```python
from build123d import *

# Parameters (mm, degrees)
F0_W     = 42
F0_H     = 17.5
F0_W_2   = 36
F0_H_2   = 11.5
F1_DEPTH = 40
F2_DEPTH = 3
F3_R     = 3
F4_R     = 2.99999


# Not quite as in the source:
# - a fillet or chamfer is up to 0.001 mm smaller than in the source, because OpenCascade refuses the exact size


with BuildPart() as f1:
    # F0 (on Top) → F1 (new body)
    with BuildSketch(Plane.XY):
        with Locations((12.1359585822, -3.1205574796)):
            Rectangle(F0_W, F0_H)
        with Locations((12.1359585822, -3.1205574796)):
            Rectangle(F0_W_2, F0_H_2, mode=Mode.SUBTRACT)
    extrude(amount=F1_DEPTH)

    # F0 (on Top) → F2 (join)
    with BuildSketch(Plane.XY):
        with Locations((12.1359585822, -3.1205574796)):
            Rectangle(F0_W, F0_H)
        with Locations((12.1359585822, -3.1205574796)):
            Rectangle(F0_W_2, F0_H_2, mode=Mode.SUBTRACT)
        with Locations((12.1359585822, -3.1205574796)):
            Rectangle(F0_W_2, F0_H_2)
    extrude(amount=-F2_DEPTH)

    # F3
    f3_edges = [f1.edges().sort_by_distance(p)[0] for p in [
        (33.135959, -11.870557, 18.5),
        (12.135959, -11.870557, -3),
        (33.135959, -3.120557, -3),
        (33.135959, 5.629443, 18.5),
        (12.135959, 5.629443, -3),
        (-8.864041, 5.629443, 18.5),
        (-8.864041, -3.120557, -3),
        (-8.864041, -11.870557, 18.5),
    ]]
    fillet(f3_edges, radius=F3_R)

    # F4 (radius 3 in the source; OpenCascade refuses exactly that, so slightly less here)
    f4_edges = [f1.edges().sort_by_distance(p)[0] for p in [
        (12.135959, 5.629443, 40),
        (-8.864041, -3.120557, 40),
        (12.135959, -11.870557, 40),
        (33.135959, -3.120557, 40),
    ]]
    fillet(f4_edges, radius=F4_R)


solid = f1.part
```
Can you work these out from the model? Positions are in its coordinate system, mm. A direction names the side the tool comes from. Coordinates: 2 decimals unless noted, no trailing zeros. Order: outer loops, then holes, each group sorted by start corner. A loop starts at its lowest first (then second) coordinate and runs counter-clockwise, first axis right, second up. Notation, with made-up numbers: (-32, 79.25) - (25, 79.25) arc R28 cw to (25, 116.25) - close; hole circle Ø10 at (59, -6.5). An arc over 180 degrees is marked (long way). Answer in a Markdown table with one row per item.
1. Suppose I cut it at A-A (z = 10.5). Please give me the cut outline in (x, y).
Reply:
| item | result |
|---|---|
| outline | (-8.86, -8.87) arc R3 ccw to (-5.86, -11.87) - (30.14, -11.87) arc R3 ccw to (33.14, -8.87) - (33.14, 2.63) arc R3 ccw to (30.14, 5.63) - (-5.86, 5.63) arc R3 ccw to (-8.86, 2.63) - close; hole (-5.86, -8.87) - (30.14, -8.87) - (30.14, 2.63) - (-5.86, 2.63) - close |
2. For pin 1 (3.5 mm diameter, centred on x = 17, y = -5, fed in from +Z), with a flat end and sliding along its axis, tell me the tip position at first contact or that it passes through.
Reply:
| item | result |
|---|---|
| pin 1 | stops at z = 0 |
3. For faces 5 (the cylindrical face through (-8.009, 4.727, 18.241)), 6 (the flat face through (-5.864, -3, 20)), which set-ups out of +Z, -Z, +X, -X, +Y, -Y let a thin tool reach every point of the face, with its end or its side?
Reply:
| item | result |
|---|---|
| face 5 | +Z, -Z, -X, +Y |
| face 6 | +Z |
4. If we mould it in two halves opening along Y, with no side actions, what happens to faces 1 (the flat face through (12, -11.871, 19)), 2 (the flat face through (12, 2.629, 20)), 3 (the flat face through (12, -3, 0)), 4 (the flat face through (33.136, -3, 19))? For each: pulls with the +Y half, pulls with the -Y half, needs draft (parallel to the pull), parting line crosses it, or undercut.
Reply:
| item | result |
|---|---|
| face 1 | pulls with the -Y half |
| face 2 | undercut |
| face 3 | undercut |
| face 4 | needs draft |
5. If I drill on line 1 along X through (y, z) = (0.5, 26.5); line 2 along Y through (x, z) = (8, 33); line 3 along Z through (x, y) = (-2, -7), over which ranges is the centre line in solid material (lowest first)?
Reply:
| item | result |
|---|---|
| line 1 | x = -8.86 to -5.86, 30.14 to 33.14 |
| line 2 | y = -11.87 to -8.87, 2.63 to 5.63 |
| line 3 | z = -3 to 0 |
